from build123d import *

# Parameters (mm, degrees)
F0_W     = 150
F0_H     = 92
F0_R     = 4
F0_R_2   = 3
F0_R_3   = 2
F1_DEPTH = 7
F2_R     = 10
F3_DEPTH = 4


with BuildPart() as f1:
    # F0 (on Top) → F1 (new body)
    with BuildSketch(Plane.XY):
        with Locations((75, 46)):
            Rectangle(F0_W, F0_H)
        with Locations((16, 10)):
            Circle(F0_R, mode=Mode.SUBTRACT)
        with Locations((15, 20)):
            Circle(F0_R_2, mode=Mode.SUBTRACT)
        with Locations((44, 10)):
            Circle(F0_R, mode=Mode.SUBTRACT)
        with Locations((55, 20)):
            Circle(F0_R_2, mode=Mode.SUBTRACT)
        with Locations((95, 20)):
            Circle(F0_R_2, mode=Mode.SUBTRACT)
        with Locations((135, 20)):
            Circle(F0_R_2, mode=Mode.SUBTRACT)
        with Locations((10, 62)):
            Circle(F0_R, mode=Mode.SUBTRACT)
        with Locations((15, 72)):
            Circle(F0_R_2, mode=Mode.SUBTRACT)
        with Locations((55, 72)):
            Circle(F0_R_2, mode=Mode.SUBTRACT)
        with Locations((95, 72)):
            Circle(F0_R_2, mode=Mode.SUBTRACT)
        with Locations((135, 72)):
            Circle(F0_R_2, mode=Mode.SUBTRACT)
        with Locations((10, 62)):
            Circle(F0_R)
        with Locations((10, 62)):
            Circle(F0_R_3, mode=Mode.SUBTRACT)
        with Locations((16, 10)):
            Circle(F0_R)
        with Locations((16, 10)):
            Circle(F0_R_3, mode=Mode.SUBTRACT)
        with Locations((44, 10)):
            Circle(F0_R)
        with Locations((44, 10)):
            Circle(F0_R_3, mode=Mode.SUBTRACT)
    extrude(amount=F1_DEPTH)

    # F2
    f2_edges = [f1.edges().sort_by_distance(p)[0] for p in [
        (0, 92, 3.5),
        (0, 0, 3.5),
        (150, 0, 3.5),
        (150, 92, 3.5),
    ]]
    fillet(f2_edges, radius=F2_R)

    # F0 (on Top) → F3 (cut)
    with BuildSketch(Plane.XY):
        with Locations((10, 62)):
            Circle(F0_R)
        with Locations((10, 62)):
            Circle(F0_R_3, mode=Mode.SUBTRACT)
        with Locations((16, 10)):
            Circle(F0_R)
        with Locations((16, 10)):
            Circle(F0_R_3, mode=Mode.SUBTRACT)
        with Locations((44, 10)):
            Circle(F0_R)
        with Locations((44, 10)):
            Circle(F0_R_3, mode=Mode.SUBTRACT)
    extrude(amount=F3_DEPTH, mode=Mode.SUBTRACT)


solid = f1.part
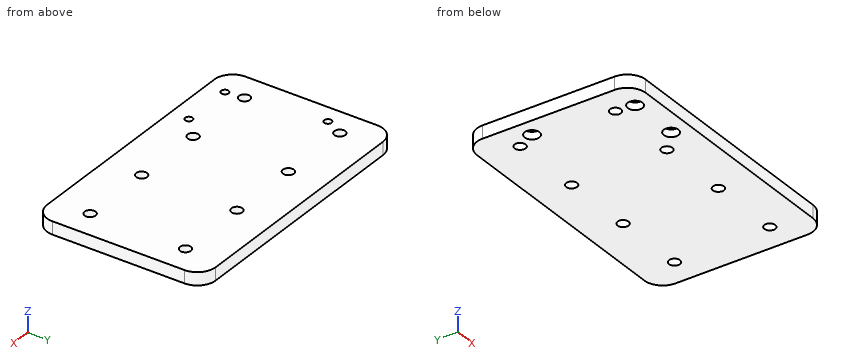
Verification items for the finished model (mm, model axes). Coordinates: 2 decimals unless noted, no trailing zeros. Loops run counter-clockwise (first coordinate to the right, second up) from the corner with the lowest first, then second, coordinate; pieces in that order, holes last. Notation, with made-up numbers: (76.5, 25.5) -> (90.5, 25.5) arc R20 ccw to (90.5, 64.5) -> close; hole circle Ø4 at (14.25, 64). An arc over 180 degrees is marked (long way). Answer as a JSON object with one key per item and string values. Group by question number.
Item 1: Sectioned sample at D-D on z = 2.75. State how many separate pieces and enclosed holes the cut face has, plus the area to 3 significant figures.
Item 2: Depth check by flat-ended pin: pin 1 (5 mm diameter, centred on x = 44, y = 10, fed in from -Z); pin 2 (5 mm diameter, centred on x = 95, y = 72, fed in from +Z). Enter the tip coordinate at first touch or a pass-through.
Item 3: Sectioned sample at B-B on x = 95. Record the boundary of the cut face in (y, z).
Item 4: Scan lines: probe 1 along Y at (x, z) = (95, 3.5); probe 2 along Y at (x, z) = (43.5, 0.75); probe 3 along X at (y, z) = (8.5, 0.75). Record each from-to range of solid material in increasing order.
Item 5: Sectioned sample at C-C on y = 62. Record the boundary of the cut face in (x, z), plus the area to 3 significant figures.
Item 6: Sectioned sample at A-A on y = 20. Record the boundary of the cut face in (x, z).
Evaluation:
{
 "1": {"separate pieces": "1", "enclosed holes": "11", "area": "13,300 mm²"},
 "2": {"pin 1": "stops at z = 4", "pin 2": "passes through"},
 "3": {"outline": "(0, 0) -> (17, 0) -> (17, 7) -> (0, 7) -> close; (23, 0) -> (69, 0) -> (69, 7) -> (23, 7) -> close; (75, 0) -> (92, 0) -> (92, 7) -> (75, 7) -> close"},
 "4": {"probe 1": "y = 0 to 17, 23 to 69, 75 to 92", "probe 2": "y = 0 to 6.03, 13.97 to 92", "probe 3": "x = 0.11 to 12.29, 19.71 to 40.29, 47.71 to 149.89"},
 "5": {"outline": "(0, 0) -> (6, 0) -> (6, 4) -> (8, 4) -> (8, 7) -> (0, 7) -> close; (12, 4) -> (14, 4) -> (14, 0) -> (150, 0) -> (150, 7) -> (12, 7) -> close", "area": "1,010 mm²"},
 "6": {"outline": "(0, 0) -> (12, 0) -> (12, 7) -> (0, 7) -> close; (18, 0) -> (52, 0) -> (52, 7) -> (18, 7) -> close; (58, 0) -> (92, 0) -> (92, 7) -> (58, 7) -> close; (98, 0) -> (132, 0) -> (132, 7) -> (98, 7) -> close; (138, 0) -> (150, 0) -> (150, 7) -> (138, 7) -> close"}
}
